from build123d import *

# Parameters (mm, degrees)
SKETCH1_R           = 9.9949
BOSS_EXTRUDE1_DEPTH = 6.9596
SKETCH2_R           = 16.51
BOSS_EXTRUDE2_DEPTH = 2.54
SKETCH5_R           = 12.7
BOSS_EXTRUDE4_DEPTH = 12.7
SKETCH6_R           = 3.96875
CUT_EXTRUDE1_DEPTH  = 22.1996


with BuildPart() as part:
    # Sketch1 → Boss-Extrude1 (new body)
    with BuildSketch(Plane.XY):
        Circle(SKETCH1_R)
    extrude(amount=BOSS_EXTRUDE1_DEPTH)

    # Sketch2 → Boss-Extrude2 (add)
    with BuildSketch(Plane.XY.offset(6.9596)):
        Circle(SKETCH2_R)
    extrude(amount=BOSS_EXTRUDE2_DEPTH)

    # Sketch5 → Boss-Extrude4 (add)
    with BuildSketch(Plane.XY.offset(9.4996)):
        Circle(SKETCH5_R)
    extrude(amount=BOSS_EXTRUDE4_DEPTH)

    # Sketch6 → Cut-Extrude1 (cut)
    with BuildSketch(Plane(origin=(0, 0, 0), x_dir=(-1, 0, 0), z_dir=(0, 0, -1))):
        Circle(SKETCH6_R)
    extrude(amount=-CUT_EXTRUDE1_DEPTH, mode=Mode.SUBTRACT)


solid = part.part
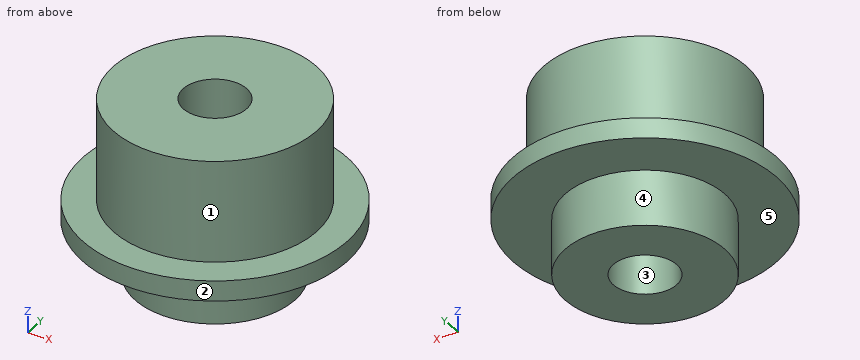
Could you check a few things on this model? Use its own coordinates, in mm. Face numbers are marked on the shaded views. A direction names the side the tool comes from. Coordinates: 2 decimals unless noted, no trailing zeros. Write each loop counter-clockwise with the first axis right and the second up, starting at its lowest first coordinate (ties: lowest second). Pieces come first, ordered by that corner, then holes. Notation, with made-up numbers: (27.5, 81.25) - (74.5, 81.25) arc R5 cw to (74.5, 89.25) - close; hole circle Ø5 at (33.25, 78). An arc over 180 degrees is marked (long way). Put each result on its own line as item: value. Start each with the question number.
Q1. I want a section at C-C on z = 19.25. Write out the boundary of the cut face in (x, y), plus the area to 3 significant figures.
Q2. Please list where these lines run through material, in increasing order: L1, parallel to Y at x = 0, z = 14; L2, parallel to Y at x = 0, z = 9; L3, parallel to Z at x = 8, y = 8.
Q3. I want a section at D-D on x = 12. Write out the boundary of the cut face in (y, z).
Q4. I want a section at A-A on x = 0. Write out the boundary of the cut face in (y, z), plus the area to 3 significant figures.
Q5. Thinking about a two-plate mould opening in Y: for the marked faces 3, 4 and 5, which applies, pulls with the +Y half, pulls with the -Y half, needs draft (parallel to the pull), parting line crosses it, or undercut?
Q6. I'm going to push flat-ended pins straight in: P1, Ø12, axis at y = 8.5, z = 4.5, coming from the -X side; P2, Ø3, axis at y = 10, z = 7, coming from the -X side; P3, Ø10, axis at x = 2, z = 18.5, coming from the +Y side; P4, Ø5, axis at x = 0, y = 0, coming from the -Z side. Where does each tip first touch, or does it pass through?
Q7. I want a section at B-B on y = -1. Write out the boundary of the cut face in (x, z), plus the area to 3 significant figures.
Q8. Which directions (+Z, -Z, +X, -X, +Y, -Y) give clear straight access to the entire face, cutting with the end or side of a thin tool? Please do the marked faces 1 and 2.
Checks:
1. outline: circle Ø25.4 at (0, 0); hole circle Ø7.94 at (0, 0)
1. area: 457 mm²
2. L1: -12.7 to -3.97, 3.97 to 12.7
2. L2: -16.51 to -3.97, 3.97 to 16.51
2. L3: 6.96 to 22.2
3. outline: (-11.34, 6.96) - (11.34, 6.96) - (11.34, 9.5) - (4.16, 9.5) - (4.16, 22.2) - (-4.16, 22.2) - (-4.16, 9.5) - (-11.34, 9.5) - close
4. outline: (-16.51, 6.96) - (-9.99, 6.96) - (-9.99, 0) - (-3.97, 0) - (-3.97, 22.2) - (-12.7, 22.2) - (-12.7, 9.5) - (-16.51, 9.5) - close; (3.97, 0) - (9.99, 0) - (9.99, 6.96) - (16.51, 6.96) - (16.51, 9.5) - (12.7, 9.5) - (12.7, 22.2) - (3.97, 22.2) - close
4. area: 369 mm²
5. face 3: undercut
5. face 4: parting line crosses it
5. face 5: needs draft
6. P1: x = -16.23
6. P2: x = -14.15
6. P3: y = 12.7
6. P4: through
7. outline: (-16.48, 6.96) - (-9.94, 6.96) - (-9.94, 0) - (-3.84, 0) - (-3.84, 22.2) - (-12.66, 22.2) - (-12.66, 9.5) - (-16.48, 9.5) - close; (3.84, 0) - (9.94, 0) - (9.94, 6.96) - (16.48, 6.96) - (16.48, 9.5) - (12.66, 9.5) - (12.66, 22.2) - (3.84, 22.2) - close
7. area: 373 mm²
8. face 1: +Z
8. face 2: +Z, -Z
